CAD build for the part. Positions are in the model's coordinates, mm. Give positions to 0.01 mm unless a question says otherwise; leave off trailing zeros. Write each loop counter-clockwise with the first axis right and the second up, starting at its lowest first coordinate (ties: lowest second). Pieces come first, ordered by that corner, then holes. Notation, with made-up numbers: (60.25, -12) - (77.25, -12) arc R13 ccw to (77.25, 7) - close; hole circle Ø11 at (60, 69). An arc over 180 degrees is marked (long way). Answer as a JSON object with one key per item and string values.
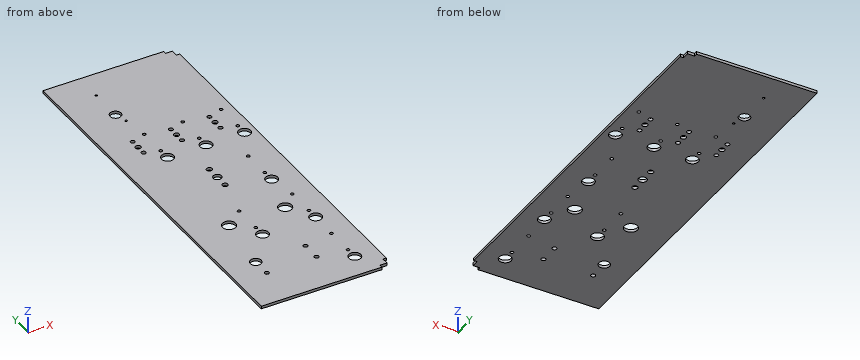
from build123d import *

# Parameters (mm, degrees)
SKETCH1_W           = 302.3362
SKETCH1_H           = 879.8306
BOSS_EXTRUDE1_DEPTH = 6.35
SKETCH2_R           = 5.08
SKETCH2_R_2         = 12.7
CUT_EXTRUDE1_DEPTH  = 931.349066226
SKETCH3_R           = 3.81
CUT_EXTRUDE2_DEPTH  = 931.349066226
SKETCH4_R           = 15.24
CUT_EXTRUDE3_DEPTH  = 931.349066226
SKETCH5_R           = 13.97
CUT_EXTRUDE4_DEPTH  = 931.349066226
SKETCH6_R           = 9.525
SKETCH6_R_2         = 6.35
CUT_EXTRUDE5_DEPTH  = 931.349066226
SKETCH7_R           = 6.35
SKETCH7_R_2         = 5.08
CUT_EXTRUDE6_DEPTH  = 931.349066226
SKETCH8_R           = 2.54
CUT_EXTRUDE7_DEPTH  = 931.349066226
SKETCH9_R           = 12.7
CUT_EXTRUDE8_DEPTH  = 931.349066226


with BuildPart() as part:
    # Sketch1 → Boss-Extrude1 (new body)
    with BuildSketch(Plane.XY):
        with Locations((151.1681, 439.9153)):
            Rectangle(SKETCH1_W, SKETCH1_H)
    extrude(amount=BOSS_EXTRUDE1_DEPTH)

    # Sketch2 → Cut-Extrude1 (cut, through all)
    with BuildSketch(Plane.XY.offset(6.35)):
        with Locations((68.3387, 97.1296)):
            Circle(SKETCH2_R)
        with Locations((68.3387, 141.6304)):
            Circle(SKETCH2_R_2)
        with Locations((183.2737, 97.1296)):
            Circle(SKETCH2_R)
        with Locations((183.2737, 141.6304)):
            Circle(SKETCH2_R)
    extrude(amount=-CUT_EXTRUDE1_DEPTH, mode=Mode.SUBTRACT)

    # Sketch3 → Cut-Extrude2 (cut, through all)
    with BuildSketch(Plane.XY.offset(6.35)):
        with Locations((250.2662, 87.122)):
            Circle(SKETCH3_R)
        with Locations((250.2662, 154.178)):
            Circle(SKETCH3_R)
        with Locations((251.5362, 247.142)):
            Circle(SKETCH3_R)
        with Locations((251.5362, 314.198)):
            Circle(SKETCH3_R)
        with Locations((128.8542, 247.142)):
            Circle(SKETCH3_R)
        with Locations((128.8542, 314.198)):
            Circle(SKETCH3_R)
        with Locations((241.6302, 407.1366)):
            Circle(SKETCH3_R)
        with Locations((241.6302, 474.1926)):
            Circle(SKETCH3_R)
        with Locations((276.9362, 577.8246)):
            Circle(SKETCH3_R)
        with Locations((276.9362, 644.8806)):
            Circle(SKETCH3_R)
        with Locations((188.0362, 577.8246)):
            Circle(SKETCH3_R)
        with Locations((188.0362, 644.8806)):
            Circle(SKETCH3_R)
        with Locations((99.1362, 577.8246)):
            Circle(SKETCH3_R)
        with Locations((99.1362, 644.8806)):
            Circle(SKETCH3_R)
    extrude(amount=-CUT_EXTRUDE2_DEPTH, mode=Mode.SUBTRACT)

    # Sketch4 → Cut-Extrude3 (cut, through all)
    with BuildSketch(Plane.XY.offset(6.35)):
        with Locations((86.4362, 280.67)):
            Circle(SKETCH4_R)
        with Locations((215.9762, 280.67)):
            Circle(SKETCH4_R)
    extrude(amount=-CUT_EXTRUDE3_DEPTH, mode=Mode.SUBTRACT)

    # Sketch5 → Cut-Extrude4 (cut, through all)
    with BuildSketch(Plane.XY.offset(6.35)):
        with Locations((250.5202, 60.245134418)):
            Circle(SKETCH5_R)
        with Locations((251.7902, 220.265134418)):
            Circle(SKETCH5_R)
        with Locations((129.1082, 220.265134418)):
            Circle(SKETCH5_R)
        with Locations((241.8842, 380.259734418)):
            Circle(SKETCH5_R)
        with Locations((277.1902, 550.947734418)):
            Circle(SKETCH5_R)
        with Locations((188.2902, 550.947734418)):
            Circle(SKETCH5_R)
        with Locations((99.3902, 550.947734418)):
            Circle(SKETCH5_R)
    extrude(amount=-CUT_EXTRUDE4_DEPTH, mode=Mode.SUBTRACT)

    # Sketch6 → Cut-Extrude5 (cut, through all)
    with BuildSketch(Plane.XY.offset(6.35)):
        with Locations((151.1427, 440.6646)):
            Circle(SKETCH6_R)
        with Locations((243.5987, 611.3526)):
            Circle(SKETCH6_R_2)
        with Locations((154.6987, 611.3526)):
            Circle(SKETCH6_R_2)
        with Locations((65.7987, 611.3526)):
            Circle(SKETCH6_R_2)
    extrude(amount=-CUT_EXTRUDE5_DEPTH, mode=Mode.SUBTRACT)

    # Sketch7 → Cut-Extrude6 (cut, through all)
    with BuildSketch(Plane.XY.offset(6.35)):
        with Locations((150.646633261, 408.918475547)):
            Circle(SKETCH7_R)
        with Locations((150.646633261, 472.410724453)):
            Circle(SKETCH7_R)
        with Locations((65.961389674, 589.137523749)):
            Circle(SKETCH7_R_2)
        with Locations((65.961389674, 633.567676251)):
            Circle(SKETCH7_R_2)
        with Locations((154.359991886, 589.137523749)):
            Circle(SKETCH7_R_2)
        with Locations((154.359991886, 633.567676251)):
            Circle(SKETCH7_R_2)
        with Locations((243.259991886, 589.137523749)):
            Circle(SKETCH7_R_2)
        with Locations((243.259991886, 633.567676251)):
            Circle(SKETCH7_R_2)
    extrude(amount=-CUT_EXTRUDE6_DEPTH, mode=Mode.SUBTRACT)

    # Sketch8 → Cut-Extrude7 (cut, through all)
    with BuildSketch(Plane.XY.offset(6.35)):
        with Locations((84.2645, 811.9745)):
            Circle(SKETCH8_R)
        with Locations((91.57335, 704.25945)):
            Circle(SKETCH8_R)
    extrude(amount=-CUT_EXTRUDE7_DEPTH, mode=Mode.SUBTRACT)

    # Sketch9 → Cut-Extrude8 (cut, through all)
    with BuildSketch(Plane.XY.offset(6.35)):
        with Locations((83.82, 733.7806)):
            Circle(SKETCH9_R)
        Polygon((278.5872, 0), (278.5872, 7.62), (294.7162, 7.62), (294.7162, 23.749), (302.3362, 23.749), (302.3362, 0), align=None)
        Polygon((302.3362, 879.8306), (302.3362, 856.0816), (294.7162, 856.0816), (294.7162, 872.2106), (278.5872, 872.2106), (278.5872, 879.8306), align=None)
    extrude(amount=-CUT_EXTRUDE8_DEPTH, mode=Mode.SUBTRACT)


solid = part.part
Item 1: Cut at B-B (z = 2). State how many separate pieces and enclosed holes the cut face has, and give its area (3 significant figures).
Entries:
{"separate pieces": "1", "enclosed holes": "42", "area": "256,000 mm2"}
Item 2: Cut at A-A (y = 280.67). Give the cut face in (x, z).
Entries:
{"outline": "(0, 0) - (71.2, 0) - (71.2, 6.35) - (0, 6.35) - close; (101.68, 0) - (200.74, 0) - (200.74, 6.35) - (101.68, 6.35) - close; (231.22, 0) - (302.34, 0) - (302.34, 6.35) - (231.22, 6.35) - close"}
Item 3: Probe line 1 (X direction, y = 282, z = 6); line 2 (X direction, y = 86.5, z = 5.25); line 3 (X direction, y = 732.5, z = 0.75). List the from-to ranges inside material, lowest first. Write a range as from..to.
Entries:
{"line 1": "0..71.25, 101.62..200.79, 231.16..302.34", "line 2": "0..246.51, 254.03..302.34", "line 3": "0..71.18, 96.46..302.34"}
Item 4: Flat gauge pins, fed straight in: P1, Ø11.5, axis at x = 183.27, y = 97.13, coming from the -Z side; P2, Ø4.5, axis at x = 251.54, y = 247.14, coming from the +Z side. Where does each tip first touch, or does it go through?
Entries:
{"P1": "z = 0", "P2": "through"}
